Autodesk Inventor part; units mm, degrees
ref_plane "YZ Plane" through (0, 0, 0) normal (1, 0, 0) x (0, 1, 0)
ref_plane "XZ Plane" through (0, 0, 0) normal (0, 1, 0) x (-1, 0, 0)
ref_plane "XY Plane" through (0, 0, 0) normal (0, 0, 1) x (1, 0, 0)
sketch "Sketch1" plane through (0, 0, 0) normal (0, 0, 1) x (1, 0, 0)
  line L0 (0, 0) -> (90, 0)
  line L1 (90, 0) -> (90, 10)
  line L2 (90, 10) -> (60, 10)
  line L3 (60, 10) -> (60, 17.5)
  line L4 (60, 17.5) -> (20, 17.5)
  line L5 (20, 17.5) -> (20, 12.5)
  line L6 (20, 12.5) -> (0, 12.5)
  line L7 (0, 12.5) -> (0, 0)
  dimension "d0" = 90
  dimension "d1" = 40
  dimension "d2" = 20
  dimension "d3" = 20
  dimension "d4" = 35
  dimension "d5" = 25
revolve "Revolution1" add sketch "Sketch1" angle 360 mid plane about axis through (0, 0, 0) along (1, 0, 0)
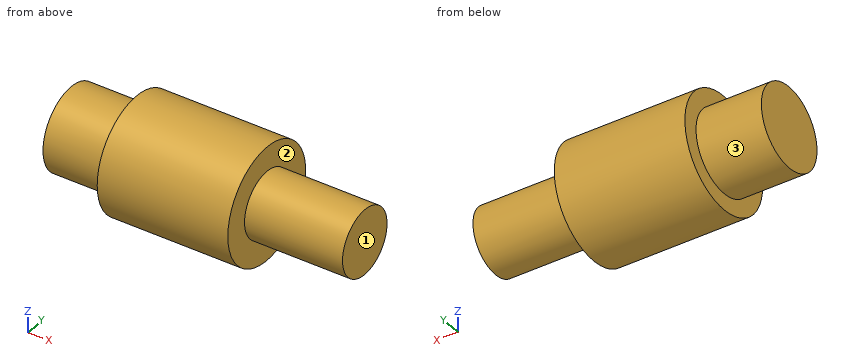
Read the model definition and answer for the solid it produces. Units are mm, in the model's axes. Face numbers are marked on the shaded views. A direction names the side the tool comes from. Round coordinates to 2 decimals unless told otherwise and drop trailing zeros. Write each loop counter-clockwise with the first axis right and the second up, starting at its lowest first coordinate (ties: lowest second). Pieces come first, ordered by that corner, then holes. Notation, with made-up numbers: (15.5, 25.25) -> (72.5, 25.25) arc R31 ccw to (72.5, 49.25) -> close; hole circle Ø6 at (-30.5, -35). An arc over 180 degrees is marked (long way). Answer in a Markdown table with one row per item. Add a question column.
1) Given P1, Ø3, axis at x = 9, y = 4, coming from the +Z side; P2, Ø2, axis at x = 65, y = -7, coming from the -Z side; P3, Ø1.5, axis at y = 13.5, z = -0.5, coming from the -X side, each flat-ended and moving along its own axis, determine where each tip first touches the part or whether it passes through.
2) Find section D-D, the plane y = 14. Determine the outline of the cut face in (x, z).
3) Which of the six approach directions +Z, -Z, +X, -X, +Y, -Y give full straight-line access (tool end or side, diameter ignored) to the marked faces 1, 2 and 3?
4) Find section A-A, the plane z = 0. Determine the outline of the cut face in (x, y).
5) Consider line 1 (X direction, y = 7.5, z = -11); line 2 (X direction, y = -5, z = -9); line 3 (Z direction, x = 37.5, y = 0). Determine where each line is inside the solid, lowest interval first.
6) Find section C-C, the plane x = 37.5. Determine the outline of the cut face in (y, z), and give its area (3 significant figures).
Findings below:
| question | item | result |
|---|---|---|
| 1 | P1 | z = 12.25 |
| 1 | P2 | z = -8 |
| 1 | P3 | x = 20 |
| 2 | outline | (20, -10.5) -> (60, -10.5) -> (60, 10.5) -> (20, 10.5) -> close |
| 3 | face 1 | +Z, -Z, +X, +Y, -Y |
| 3 | face 2 | +X |
| 3 | face 3 | -X |
| 4 | outline | (0, -12.5) -> (20, -12.5) -> (20, -17.5) -> (60, -17.5) -> (60, -10) -> (90, -10) -> (90, 10) -> (60, 10) -> (60, 17.5) -> (20, 17.5) -> (20, 12.5) -> (0, 12.5) -> close |
| 5 | line 1 | 20 to 60 |
| 5 | line 2 | 0 to 60 |
| 5 | line 3 | -17.5 to 17.5 |
| 6 | outline | circle Ø35 at (0, 0) |
| 6 | area | 962 mm² |
